Autodesk Inventor part; units mm, degrees
ref_plane "XY Plane" through (0, 0, 0) normal (0, 0, 1) x (1, 0, 0)
sketch "スケッチ1" plane through (0, 0, 0) normal (0, 0, 1) x (1, 0, 0)
  arc A0 (0, 35) -> (0, -35) centre (0, 0) ccw
  line L0 (0, 35) -> (0, -35)
  dimension "d0" = 70
revolve "回転1" add sketch "スケッチ1" angle 360 about axis through (0, 35, 0) along (0, -1, 0)
sketch "スケッチ2" plane through (0, 0, 0) normal (1, 0, 0) x (0, 1, 0)
  circle A0 centre (0, 0) radius 20
  dimension "d2" = 40
extrude "押し出し1" cut sketch "スケッチ2" along normal mid plane 100
sketch "スケッチ4" plane through (0, 0, 0) normal (0, 1, 0) x (-1, 0, 0)
  circle A0 centre (0, 0) radius 15
  dimension "d8" = 30
extrude "押し出し3" add sketch "スケッチ4" along normal mid plane 75
properties part number "FootR"
The listing builds one solid part. Answer for the finished solid, in the listing's coordinates (mm). A direction names the side the tool comes from. Coordinates: 2 decimals unless noted, no trailing zeros. Write each loop counter-clockwise with the first axis right and the second up, starting at its lowest first coordinate (ties: lowest second). Pieces come first, ordered by that corner, then holes. Notation, with made-up numbers: M -15.75,34.5 L -9.75,34.5 A11 cw -9.75,49.5 Z; hole C 77,25.25 d5. An arc over 180 degrees is marked long. Use a Markdown table: item, result. Add a question column.
1. Section A-A (y = 0) is taken. Give the vertices of the cut face in (x, z), plus the area to 3 significant figures.
2. Section C-C (z = -3) is taken. Give the vertices of the cut face in (x, y), plus the area to 3 significant figures.
3. For a pull along Y with two mould halves and no side action, classify faces 1 (the flat face through (0, 37.5, 0)), 2 (the cylindrical face through (0.402, 10.752, 16.864)), 3 (the cylindrical face through (14.985, -34.52, 0.66)) as +Y half, -Y half, draft (parallel to the pull), parting line (faces both ways), or undercut.
4. Which of the six approach directions +Z, -Z, +X, -X, +Y, -Y give full straight-line access (tool end or side, diameter ignored) to faces 4 (the cylindrical face through (-6.92, 0.28, -13.31)), 5 (the cylindrical face through (14.985, 34.52, -0.66)), 6 (the flat face through (0, -37.5, 0))?
5. Straight lines are drawn through the part: line 1 along Z through (x, y) = (12, 0); line 2 along Z through (x, y) = (-3, -1.5); line 3 along Y through (x, z) = (16, 0). For each, find the intervals that lie inside material, in ascending order. Write a range as [from, to].
6. Section D-D (x = -21) is taken. Give the vertices of the cut face in (y, z).
7. Given P1, Ø6, axis at x = -3, z = 20.5, coming from the -Y side; P2, Ø10, axis at x = -19.5, y = -3, coming from the +Z side; P3, Ø1.5, axis at x = 5, y = -26, coming from the -Z side, each flat-ended and moving along its own axis, determine where each tip first touches the part or whether it passes through.
8. Section B-B (x = -5.5) is taken. Give the vertices of the cut face in (y, z).
Data:
| question | item | result |
|---|---|---|
| 1 | outline | M -28.72,-20 A35 ccw 28.72,-20 Z; M -28.72,20 L 28.72,20 A35 ccw Z; C 0,0 d30 |
| 1 | area | 1,920 mm2 |
| 2 | outline | M -28.72,-19.77 A34.87 ccw -14.7,-31.62 L -14.7,-37.5 L 14.7,-37.5 L 14.7,-31.62 A34.87 ccw 28.72,-19.77 L 14.7,-19.77 L 14.7,19.77 L 28.72,19.77 A34.87 ccw 14.7,31.62 L 14.7,37.5 L -14.7,37.5 L -14.7,31.62 A34.87 ccw -28.72,19.77 L -14.7,19.77 L -14.7,-19.77 Z |
| 2 | area | 2,600 mm2 |
| 3 | face 1 | +Y half |
| 3 | face 2 | undercut |
| 3 | face 3 | draft |
| 4 | face 4 | none |
| 4 | face 5 | +Y |
| 4 | face 6 | +Z, -Z, +X, -X, -Y |
| 5 | line 1 | z = [-32.88, -20], [-9, 9], [20, 32.88] |
| 5 | line 2 | z = [-34.84, -19.94], [-14.7, 14.7], [19.94, 34.84] |
| 5 | line 3 | y = [-31.13, -20], [20, 31.13] |
| 6 | outline | C 0,0 d56; hole C 0,0 d40 |
| 7 | P1 | stops at y = -30.18 |
| 7 | P2 | stops at z = 31.75 |
| 7 | P3 | stops at z = -23.73 |
| 8 | outline | M -37.5,-13.96 L -31.62,-13.96 A34.57 ccw 31.62,-13.96 L 37.5,-13.96 L 37.5,13.96 L 31.62,13.96 A34.57 ccw -31.62,13.96 L -37.5,13.96 Z; hole M -14.33,-13.96 A20 ccw 14.33,-13.96 Z; hole M -14.33,13.96 L 14.33,13.96 A20 ccw Z |
